from build123d import *

# Parameters (mm, degrees)
SKETCH1_R               = 30.55
BOSS_EXTRUDE1_DEPTH     = 20.32
SKETCH2_R               = 25.404
CUT_EXTRUDE1_DEPTH      = 13
SKETCH3_R               = 20
CUT_EXTRUDE2_DEPTH      = 21.32
FILLET1_R               = 1
FILLET2_R               = 1
SKETCH4_W               = 27.244453354
SKETCH4_H               = 24.319072788
CUT_EXTRUDE3_DEPTH      = 31.55
CUT_EXTRUDE3_DEPTH_BACK = 31.55


with BuildPart() as part:
    # Sketch1 → Boss-Extrude1 (new body)
    with BuildSketch(Plane(origin=(0, 0, 0), x_dir=(1, 0, 0), z_dir=(0, 1, 0))):
        Circle(SKETCH1_R)
    extrude(amount=BOSS_EXTRUDE1_DEPTH)

    # Sketch2 → Cut-Extrude1 (cut)
    with BuildSketch(Plane.XZ):
        Circle(SKETCH2_R)
    extrude(amount=-CUT_EXTRUDE1_DEPTH, mode=Mode.SUBTRACT)

    # Sketch3 → Cut-Extrude2 (cut, through all)
    with BuildSketch(Plane(origin=(0, 20.32, 0), x_dir=(1, 0, 0), z_dir=(0, 1, 0))):
        Circle(SKETCH3_R)
    extrude(amount=-CUT_EXTRUDE2_DEPTH, mode=Mode.SUBTRACT)

    # Fillet1
    fillet1_edges = [part.edges().sort_by_distance(p)[0] for p in [
        (-25.404, 0, 0),
    ]]
    fillet(fillet1_edges, radius=FILLET1_R)

    # Fillet2
    fillet2_edges = [part.edges().sort_by_distance(p)[0] for p in [
        (-20, 13, 0),
    ]]
    fillet(fillet2_edges, radius=FILLET2_R)

    # Sketch4 → Cut-Extrude3 (cut, two sides)
    with BuildSketch(Plane.XY) as cut_extrude3_sk:
        with Locations((-0.856929661, 18.03488809)):
            Rectangle(SKETCH4_W, SKETCH4_H)
    extrude(amount=CUT_EXTRUDE3_DEPTH, mode=Mode.SUBTRACT)
    extrude(cut_extrude3_sk.sketch, amount=-CUT_EXTRUDE3_DEPTH_BACK, mode=Mode.SUBTRACT)


solid = part.part
The listing builds one solid part. Answer for the finished solid, in the listing's coordinates (mm). A direction names the side the tool comes from. Round coordinates to 2 decimals unless told otherwise and drop trailing zeros. Order: outer loops, then holes, each group sorted by start corner. A loop starts at its lowest first (then second) coordinate and runs counter-clockwise, first axis right, second up. Notation, with made-up numbers: (73.25, 70.25) -> (119.25, 70.25) arc R7 cw to (119.25, 74.25) -> close; hole circle Ø7 at (66.5, 51). An arc over 180 degrees is marked (long way). Put each result on its own line as item: value.
Q1. Section B-B, the plane z = 0 is taken. Write down the section's boundary in (x, y), and give its area (3 significant figures).
Results list:
outline: (-30.55, 0) -> (-26.4, 0) arc R1 ccw to (-25.4, 1) -> (-25.4, 13) -> (-21, 13) arc R1 ccw to (-20, 14) -> (-20, 20.32) -> (-30.55, 20.32) -> close; (20, 14) arc R1 ccw to (21, 13) -> (25.4, 13) -> (25.4, 1) arc R1 ccw to (26.4, 0) -> (30.55, 0) -> (30.55, 20.32) -> (20, 20.32) -> close
area: 287 mm^2
Q2. Section A-A, the plane y = 9 is taken. Write down the section's boundary in (x, z), and give its area (3 significant figures).
Results list:
outline: (-14.48, -26.9) -> (-14.48, -20.87) arc R25.4 cw to (-14.48, 20.87) -> (-14.48, 26.9) arc R30.55 ccw to start; (12.77, -27.76) arc R30.55 ccw to (12.77, 27.76) -> (12.77, 21.96) arc R25.4 cw to (12.77, -21.96) -> close
area: 611 mm^2
Q3. Section D-D, the plane y = 15 is taken. Write down the section's boundary in (x, z).
Results list:
outline: (-14.48, -26.9) -> (-14.48, -13.8) arc R20 cw to (-14.48, 13.8) -> (-14.48, 26.9) arc R30.55 ccw to start; (12.77, -27.76) arc R30.55 ccw to (12.77, 27.76) -> (12.77, 15.4) arc R20 cw to (12.77, -15.4) -> close
Q4. Consider line 1 along Z through (x, y) = (0, 4); line 2 along Y through (x, z) = (-8.5, -25). Determine where each line is inside the solid, lowest interval first.
Results list:
line 1: -30.55 to -25.4, 25.4 to 30.55
line 2: 0 to 5.88
Q5. Section C-C, the plane x = 0 is taken. Write down the section's boundary in (y, z).
Results list:
outline: (0, -30.55) -> (5.88, -30.55) -> (5.88, -25.4) -> (1, -25.4) arc R1 ccw to (0, -26.4) -> close; (0, 26.4) arc R1 ccw to (1, 25.4) -> (5.88, 25.4) -> (5.88, 30.55) -> (0, 30.55) -> close
Q6. Which of the six approach directions +Z, -Z, +X, -X, +Y, -Y give full straight-line access (tool end or side, diameter ignored) to faces 1 (the flat face through (22, 20.32, 0)), 2 (the cylindrical face through (-3.307, 5.583, 25.188)), 3 (the flat face through (-14.479, 15, 22)), 4 (the cylindrical face through (20, 17, 0))?
Results list:
face 1: +Z, -Z, +X, -X, +Y
face 2: -Y
face 3: +Z, -Z, +Y
face 4: +Y, -Y
Q7. Each of these flat-tipped pins is pushed along its axis until it touches: P1, Ø8, axis at x = 1.5, y = 3.5, coming from the -Z side; P2, Ø1.5, axis at x = 16, y = 12.5, coming from the +Z side; P3, Ø3, axis at x = 2, z = 27.5, coming from the +Y side. Where does it stop, or does it pass through?
Results list:
P1: z = -30.55
P2: z = 26.47
P3: y = 5.88
Q8. Determine the mould class of faces 5 (the flat face through (-14.479, 15, -22)), 6 (the cylindrical face through (-20, 17, 0)), 7 (the cylindrical face through (29.14, 10.02, -9.18)) for opening direction Z: pulls with the +Z half, pulls with the -Z half, needs draft (parallel to the pull), parting line crosses it, or undercut.
Results list:
face 5: needs draft
face 6: undercut
face 7: parting line crosses it
